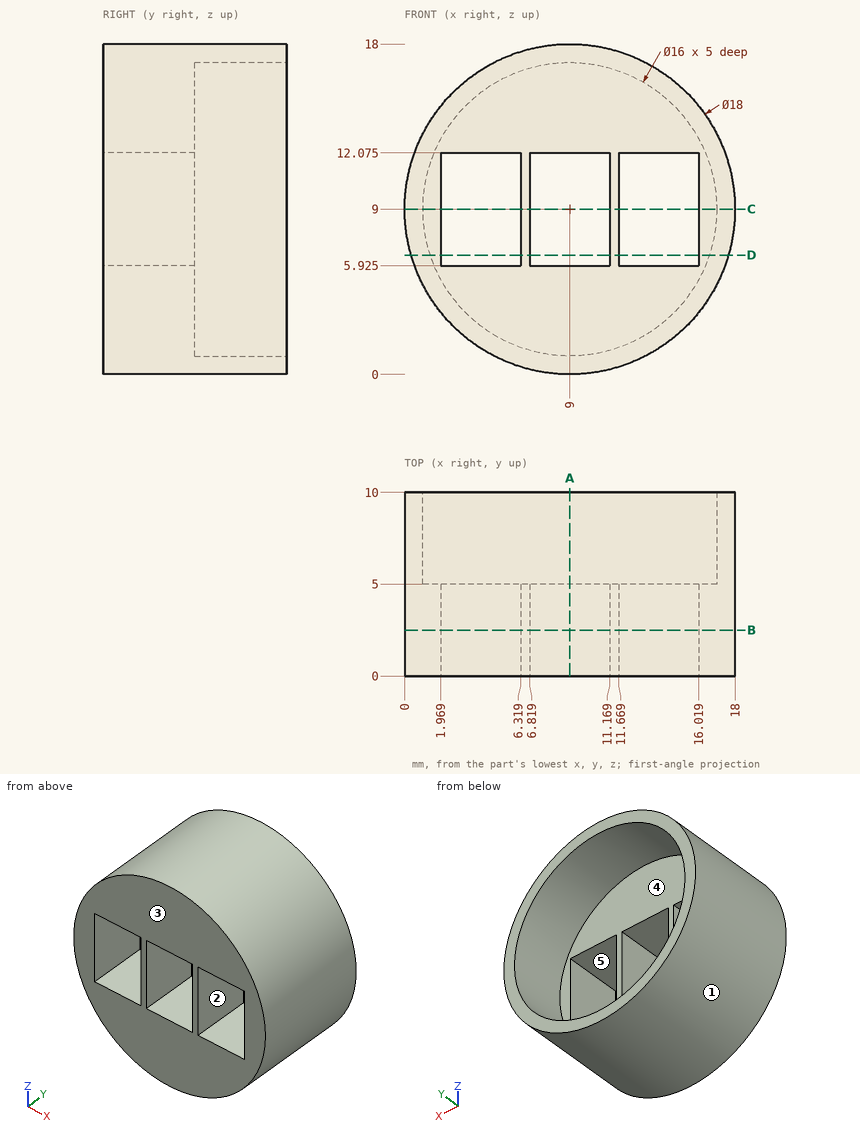
Design review of the part shown in the three views and the two pictorial views. Dimensions are in mm from the part's minimum x, y and z. A direction names the side the tool comes from. Round coordinates to 2 decimals unless told otherwise and drop trailing zeros. Loops run counter-clockwise (first coordinate to the right, second up) from the corner with the lowest first, then second, coordinate; pieces in that order, holes last. Notation, with made-up numbers: (28.5, 17.5) - (46.5, 17.5) arc R21 ccw to (46.5, 35.5) - close; hole circle Ø8 at (-34.75, 80). An arc over 180 degrees is marked (long way). Use one line per item in the form item = value.
1) Clearance check with flat-ended pins moving along their axes: P1, Ø5, axis at x = 3, y = 1.5, coming from the -Z side; P2, Ø5, axis at x = 3.5, y = 1.5, coming from the +Z side; P3, Ø5, axis at x = 14.5, y = 2.5, coming from the -Z side. State where each tip first meets the part, or that it passes through.
Solutions:
P1 = 0.71
P2 = 17.49
P3 = 0.51
2) Mouldability with a two-part tool opening along Z and no side actions: class the marked faces 1, 2 and 3 as pulls with the +Z half, pulls with the -Z half, needs draft (parallel to the pull), parting line crosses it, or undercut.
Solutions:
face_1 = parting line crosses it
face_2 = undercut
face_3 = needs draft
3) We need section B-B on y = 2.5. Write out the cut boundary in (x, z) (3 decimals), then the cut area to 3 significant figures.
Solutions:
outline = circle Ø18 at (9, 9); hole (1.969, 5.925) - (6.319, 5.925) - (6.319, 12.075) - (1.969, 12.075) - close; hole (6.819, 5.925) - (11.169, 5.925) - (11.169, 12.075) - (6.819, 12.075) - close; hole (11.669, 5.925) - (16.019, 5.925) - (16.019, 12.075) - (11.669, 12.075) - close
area = 174 mm2
4) We need section C-C on z = 9. Write out the cut boundary in (x, y).
Solutions:
outline = (0, 0) - (1.97, 0) - (1.97, 5) - (1, 5) - (1, 10) - (0, 10) - close; (6.32, 0) - (6.82, 0) - (6.82, 5) - (6.32, 5) - close; (11.17, 0) - (11.67, 0) - (11.67, 5) - (11.17, 5) - close; (16.02, 0) - (18, 0) - (18, 10) - (17, 10) - (17, 5) - (16.02, 5) - close
5) Tool access review of the marked faces 4 and 5: name each direction out of +Z, -Z, +X, -X, +Y, -Y from which nothing blocks a thin tool from reaching the whole face with its end or side.
Solutions:
face_4 = +Y
face_5 = +Y, -Y
6) We need section D-D on z = 6.5. Write out the cut boundary in (x, y), then the cut area to 3 significant figures.
Solutions:
outline = (0.35, 0) - (1.97, 0) - (1.97, 5) - (1.4, 5) - (1.4, 10) - (0.35, 10) - close; (6.32, 0) - (6.82, 0) - (6.82, 5) - (6.32, 5) - close; (11.17, 0) - (11.67, 0) - (11.67, 5) - (11.17, 5) - close; (16.02, 0) - (17.65, 0) - (17.65, 10) - (16.6, 10) - (16.6, 5) - (16.02, 5) - close
area = 31.7 mm2
7) Wall thickness on probe 1 along X at (y, z) = (7.95, 9); probe 2 along Y at (x, z) = (5, 13.25): over which ranges is each line inside the solid? List them lowest first.
Solutions:
probe_1 = 0 to 1, 17 to 18
probe_2 = 0 to 5
8) We need section A-A on x = 9. Write out the cut boundary in (y, z) (3 decimals).
Solutions:
outline = (0, 0) - (10, 0) - (10, 1) - (5, 1) - (5, 5.925) - (0, 5.925) - close; (0, 12.075) - (5, 12.075) - (5, 17) - (10, 17) - (10, 18) - (0, 18) - close
